Here's how the part is built. I have some questions about the finished solid (model axes, mm). Face numbers are marked on the shaded views. A direction names the side the tool comes from. Round coordinates to 2 decimals unless told otherwise and drop trailing zeros. Loops run counter-clockwise (first coordinate to the right, second up) from the corner with the lowest first, then second, coordinate; pieces in that order, holes last. Notation, with made-up numbers: M -33.5,73 L -9.5,73 A22 cw -9.5,103 Z; hole C 70,-7 d7. An arc over 180 degrees is marked long. Answer as a JSON object with one key per item and string values.
from build123d import *

# Parameters (mm, degrees)
SKETCH1_R             = 4
MAIN_DEPTH            = 6
SCREWBALLDRIVER_DEPTH = 15
SKETCH3_W             = 2.9
SKETCH3_H             = 10
MAKERBEAMRAIL_DEPTH   = 7.5
SKETCH4_R             = 1.5
MAKERBEAMHOLE_DEPTH   = 15


with BuildPart() as part:
    # Sketch1 → Main (new body, symmetric)
    with BuildSketch(Plane.XY):
        with BuildLine():
            Line((-20, 6.5), (20, 6.5))
            ThreePointArc((20, 6.5), (26.5, 0), (20, -6.5))
            Line((20, -6.5), (-20, -6.5))
            ThreePointArc((-20, -6.5), (-26.5, 0), (-20, 6.5))
        make_face()
        with Locations((-20, 0)):
            Circle(SKETCH1_R, mode=Mode.SUBTRACT)
        with Locations((20, 0)):
            Circle(SKETCH1_R, mode=Mode.SUBTRACT)
    extrude(amount=MAIN_DEPTH, both=True)

    # Sketch2 → ScrewBallDriver (cut, symmetric)
    with BuildSketch(Plane(origin=(0, 0, 0), x_dir=(0, 0, -1), z_dir=(1, 0, 0))):
        with BuildLine():
            Line((-6, 6.5), (-6, -6.5))
            ThreePointArc((-6, -6.5), (-5.140215409, 0), (-6, 6.5))
        make_face()
    extrude(amount=SCREWBALLDRIVER_DEPTH, both=True, mode=Mode.SUBTRACT)

    # Sketch3 → MakerBeamRail (add)
    with BuildSketch(Plane(origin=(0, 0, 0), x_dir=(1, 0, 0), z_dir=(0, 1, 0))):
        with Locations((0, 1)):
            Rectangle(SKETCH3_W, SKETCH3_H)
    extrude(amount=MAKERBEAMRAIL_DEPTH)

    # Sketch4 → MakerBeamHole (cut, through all)
    with BuildSketch(Plane(origin=(0, 7.5, 0), x_dir=(1, 0, 0), z_dir=(0, 1, 0))):
        Circle(SKETCH4_R)
    extrude(amount=-MAKERBEAMHOLE_DEPTH, mode=Mode.SUBTRACT)


solid = part.part
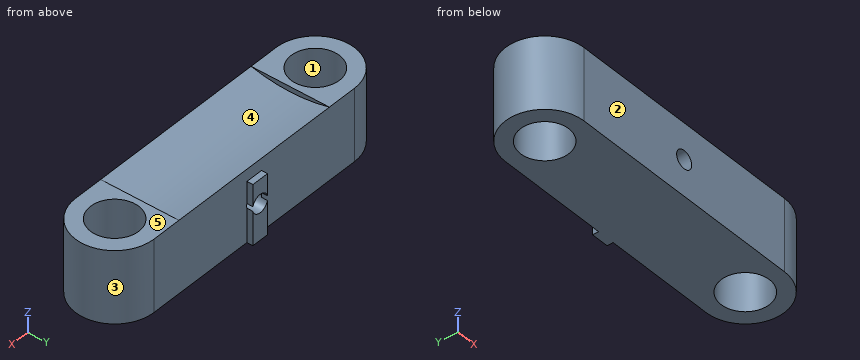
Item 1: I want a section at D-D on y = 4.5. List the corners of the cut face in (x, z) for me, plus the area to 3 significant figures.
Solution:
{"outline": "M -24.69,-6 L 24.69,-6 L 24.69,6 L 15,6 L 15,5.55 L -15,5.55 L -15,6 L -24.69,6 Z; hole C 0,0 d3", "area": "572 mm2"}
Item 2: We'd pull the mould along X, two halves only. Please class the marked faces 1, 2 and 3: +X half, -X half, draft (parallel to the pull), parting line (faces both ways), or undercut.
Solution:
{"face 1": "undercut", "face 2": "draft", "face 3": "+X half"}
Item 3: For P1, Ø7, axis at x = 20, y = 0, coming from the +Z side; P2, Ø0.5, axis at y = 7, z = -3.5, coming from the -X side; P3, Ø0.5, axis at y = 7, z = 2, coming from the +X side; P4, Ø2, axis at x = -18.5, z = 1, coming from the +Y side, each with a flat end and sliding along its axis, tell me the tip position at first contact or that it passes through.
Solution:
{"P1": "passes through", "P2": "stops at x = -1.45", "P3": "stops at x = 1.45", "P4": "stops at y = 6.5"}
Item 4: I want a section at C-C on z = 2.5. List the corners of the cut face in (x, y) for me, plus the area to 3 significant figures.
Solution:
{"outline": "M -20,-6.5 L 20,-6.5 A6.5 ccw 20,6.5 L 1.45,6.5 L 1.45,7.5 L -1.45,7.5 L -1.45,6.5 L -20,6.5 A6.5 ccw Z; hole C -20,0 d8; hole C 20,0 d8", "area": "555 mm2"}
Item 5: For the marked faces 4 and 5, which set-ups out of +Z, -Z, +X, -X, +Y, -Y let a thin tool reach every point of the face, with its end or its side?
Solution:
{"face 4": "+Z", "face 5": "+Z, +X, -X, +Y, -Y"}
Item 6: I want a section at A-A on y = 0. List the corners of the cut face in (x, z) for me.
Solution:
{"outline": "M -26.5,-6 L -24,-6 L -24,6 L -26.5,6 Z; M -16,-6 L 16,-6 L 16,6 L 15,6 L 15,5.14 L -15,5.14 L -15,6 L -16,6 Z; M 24,-6 L 26.5,-6 L 26.5,6 L 24,6 Z; hole C 0,0 d3"}
Item 7: If I drill on L1, parallel to X at y = -1.25, z = -5.5; L2, parallel to X at y = 0.75, z = -3.75; L3, parallel to Y at x = 20, z = 2, over which ranges is the centre line in solid material (lowest first)? Write a range as from..to.
Solution:
{"L1": "x = -26.38..-23.8, -16.2..16.2, 23.8..26.38", "L2": "x = -26.46..-23.93, -16.07..16.07, 23.93..26.46", "L3": "y = -6.5..-4, 4..6.5"}
Item 8: I want a section at B-B on x = 0. List the corners of the cut face in (y, z) for me, plus the area to 3 significant figures.
Solution:
{"outline": "M -6.5,-6 L 7.5,-6 L 7.5,-1.5 L -6.5,-1.5 Z; M -6.5,1.5 L 7.5,1.5 L 7.5,4 L 6.5,4 L 6.5,6 A25 cw -6.5,6 Z", "area": "117 mm2"}
